from build123d import *

# Parameters (mm, degrees)
SKETCH1_R                = 5
BOSS_EXTRUDE1_DEPTH      = 31
BOSS_EXTRUDE2_DEPTH      = 10
BOSS_EXTRUDE2_DEPTH_BACK = 41
SKETCH2_R                = 4
SKETCH3_R                = 1.75
CUT_EXTRUDE1_DEPTH       = 1.5
CUT_EXTRUDE2_START       = -1.5
SKETCH4_R                = 1.75
CUT_EXTRUDE2_DEPTH       = 1.5


with BuildPart() as part:
    # Sketch1 → Boss-Extrude1 (new body)
    with BuildSketch(Plane(origin=(0, 0, 0), x_dir=(1, 0, 0), z_dir=(0, 1, 0))):
        with Locations(Location((0, 0, 0), (0, 0, 270))):
            Circle(SKETCH1_R)
    extrude(amount=BOSS_EXTRUDE1_DEPTH)

    # Sketch2 → Boss-Extrude2 (add, two sides: drawn at the far end of the back side and taken through both)
    with BuildSketch(Plane(origin=(0, 31, 0), x_dir=(1, 0, 0), z_dir=(0, 1, 0)).offset(-BOSS_EXTRUDE2_DEPTH_BACK)):
        with Locations(Location((0, 0, 0), (0, 0, 270))):
            Circle(SKETCH2_R)
    extrude(amount=BOSS_EXTRUDE2_DEPTH + BOSS_EXTRUDE2_DEPTH_BACK)

    # Sketch3 → Cut-Extrude1 (cut)
    with BuildSketch(Plane.XZ.offset(10)):
        with Locations(Location((0, 0, 0), (0, 0, 270))):
            Circle(SKETCH3_R)
    extrude(amount=-CUT_EXTRUDE1_DEPTH, mode=Mode.SUBTRACT)

    # Sketch4 → Cut-Extrude2 (cut)
    with BuildSketch(Plane(origin=(0, 41, 0), x_dir=(1, 0, 0), z_dir=(0, 1, 0)).offset(CUT_EXTRUDE2_START)):
        with Locations(Location((0, 0, 0), (0, 0, 90))):
            Circle(SKETCH4_R)
    extrude(amount=CUT_EXTRUDE2_DEPTH, mode=Mode.SUBTRACT)


solid = part.part
Input: part model. Units: mm. Frame: model coordinates. A direction names the side the tool comes from. Coordinates: 2 decimals unless noted, no trailing zeros. Write each loop counter-clockwise with the first axis right and the second up, starting at its lowest first coordinate (ties: lowest second). Pieces come first, ordered by that corner, then holes. Notation, with made-up numbers: M 23,27.5 L 29,27.5 A26 cw 29,53.5 Z; hole C 8.25,6.5 d11. An arc over 180 degrees is marked long. Answer as a JSON object with one key per item and string values. Group by question number.
(1) Contact query for flat-ended pins moving along their axis: P1, Ø2, axis at y = 6, z = -1.5, coming from the -X side; P2, Ø3, axis at y = 24, z = 3, coming from the +X side; P3, Ø2, axis at x = 2.5, y = 10.5, coming from the +Z side. Output: stop coordinate, or through.
(2) Section A-A on x = 0. Output: boundary loops of the cut face in (y, z), plus the area to 4 significant figures.
(3) Mould query, pull axis Z, two halves, no side actions, for faces 1 (the face through (-1.71, -9.26, 0.38)), 2 (the face through (-1, 41, 2)), 3 (the face through (-3.905, 35.93, -0.867)). Classes: pulls with the +Z half, pulls with the -Z half, needs draft (parallel to the pull), parting line crosses it, or undercut.
(4) Section D-D on x = 3. Output: boundary loops of the cut face in (y, z), plus the area to 3 significant figures.
(5) Section B-B on z = 0. Output: boundary loops of the cut face in (x, y).
(6) Ray query, line 1 along X through (y, z) = (40.05, 0); line 2 along Y through (x, z) = (3.5, 2); line 3 along X through (y, z) = (4.5, -3). Return the intervals inside material, ascending. Write a range as [from, to].
(7) Section C-C on y = 6.5. Output: boundary loops of the cut face in (x, z), plus the area to 3 significant figures.
(8) Set-up query: faces 4 (the face through (0, -8.5, 0)), 5 (the face through (-4.88, 15.28, -1.08)), 6 (the face through (0, 39.5, 0)). Return all of +Z, -Z, +X, -X, +Y, -Y with unobstructed straight access to the full face (end or side cutting, diameter ignored); none if empty.
Result set:
{
 "1": {"P1": "stops at x = -4.97", "P2": "stops at x = 4.77", "P3": "stops at z = 4.77"},
 "2": {"outline": "M -10,-4 L 0,-4 L 0,-5 L 31,-5 L 31,-4 L 41,-4 L 41,-1.75 L 39.5,-1.75 L 39.5,1.75 L 41,1.75 L 41,4 L 31,4 L 31,5 L 0,5 L 0,4 L -10,4 L -10,1.75 L -8.5,1.75 L -8.5,-1.75 L -10,-1.75 Z", "area": "459.5 mm2"},
 "3": {"face 1": "undercut", "face 2": "needs draft", "face 3": "parting line crosses it"},
 "4": {"outline": "M -10,-2.65 L 0,-2.65 L 0,-4 L 31,-4 L 31,-2.65 L 41,-2.65 L 41,2.65 L 31,2.65 L 31,4 L 0,4 L 0,2.65 L -10,2.65 Z", "area": "354 mm2"},
 "5": {"outline": "M -5,0 L -4,0 L -4,-10 L -1.75,-10 L -1.75,-8.5 L 1.75,-8.5 L 1.75,-10 L 4,-10 L 4,0 L 5,0 L 5,31 L 4,31 L 4,41 L 1.75,41 L 1.75,39.5 L -1.75,39.5 L -1.75,41 L -4,41 L -4,31 L -5,31 Z"},
 "6": {"line 1": "x = [-4, -1.75], [1.75, 4]", "line 2": "y = [0, 31]", "line 3": "x = [-4, 4]"},
 "7": {"outline": "C 0,0 d10", "area": "78.5 mm2"},
 "8": {"face 4": "-Y", "face 5": "+Y, -Y", "face 6": "+Y"}
}
